Can you work these out from the model? Positions are in its coordinate system, mm. Face numbers are marked on the shaded views. A direction names the side the tool comes from. Coordinates: 2 decimals unless noted, no trailing zeros. Order: outer loops, then holes, each group sorted by start corner. A loop starts at its lowest first (then second) coordinate and runs counter-clockwise, first axis right, second up. Notation, with made-up numbers: (56, 0.25) - (64, 0.25) arc R21 cw to (64, 31.25) - close; hole circle Ø1 at (68, -7.5). An arc over 180 degrees is marked (long way). Return JSON: item names as keys, results as strings. Group by question number.
1) If I drill on line 1 along X through (y, z) = (0.85, 2.5); line 2 along Z through (x, y) = (12.75, 6.5); line 3 along Y through (x, z) = (11.5, 7.75), over which ranges is the centre line in solid material (lowest first)?
2) Imagine slicing it at D-D (y = 4.5). Write out the boundary of the cut face in (x, z), and give its area (3 significant figures).
3) If we mould it in two halves opening along X, with no side actions, what happens to the marked faces 3, 4 and 5? For each: pulls with the +X half, pulls with the -X half, needs draft (parallel to the pull), parting line crosses it, or undercut.
4) Imagine slicing it at C-C (x = 12.5). Write out the boundary of the cut face in (y, z).
5) Which directions (+Z, -Z, +X, -X, +Y, -Y) give clear straight access to the entire face, cutting with the end or side of a thin tool? Please do the marked faces 1 and 2.
6) Imagine slicing it at A-A (z = 2.5). Write out the boundary of the cut face in (x, y).
7) For pin 1 Ø6.5 at (x, z) = (10.5, 5.5) entering from -Y; pin 2 Ø7.5 at (x, y) = (8.5, 6) entering from -Z; pin 3 Ø0.5 at (y, z) = (-0.5, 11) entering from +X; pin 4 Ø2.5 at (x, z) = (15.5, 2.5) entering from -Y, each with a flat end and sliding along its axis, tell me the tip position at first contact or that it passes through.
8) Imagine slicing it at B-B (x = 15.5). Write out the boundary of the cut face in (y, z).
```python
from build123d import *

# Parameters (mm, degrees)
SKETCH_1_W      = 18
SKETCH_1_H      = 13
SKETCH_1_R      = 1.5
EXTRUDE_1_DEPTH = 1.6
SKETCH_2_W      = 15
SKETCH_2_H      = 1.5
EXTRUDE_2_DEPTH = 1
SKETCH_3_W      = 15.814161569
SKETCH_3_H      = 0.898910236
EXTRUDE_3_DEPTH = 15


with BuildPart() as part:
    # 草图1 → 凸台-拉伸1 (new body)
    with BuildSketch(Plane(origin=(0, 0, 0), x_dir=(1, 0, 0), z_dir=(0, 1, 0))):
        with Locations((9, -6.5)):
            Rectangle(SKETCH_1_W, SKETCH_1_H)
        with Locations(Location((2.5, -2.5, 0), (0, 0, 270))):
            Circle(SKETCH_1_R, mode=Mode.SUBTRACT)
        with Locations(Location((15.5, -2.5, 0), (0, 0, 270))):
            Circle(SKETCH_1_R, mode=Mode.SUBTRACT)
    extrude(amount=EXTRUDE_1_DEPTH)

    # 草图2 → 凸台-拉伸2 (add)
    with BuildSketch(Plane.XZ):
        with Locations((9, 11.25)):
            Rectangle(SKETCH_2_W, SKETCH_2_H)
    extrude(amount=EXTRUDE_2_DEPTH)

    # 草图3 → 凸台-拉伸3 (add)
    with BuildSketch(Plane(origin=(0, 1.6, 0), x_dir=(1, 0, 0), z_dir=(0, 1, 0))):
        with Locations((8.933414057, -11.968370606)):
            Rectangle(SKETCH_3_W, SKETCH_3_H)
    extrude(amount=EXTRUDE_3_DEPTH)


solid = part.part
```
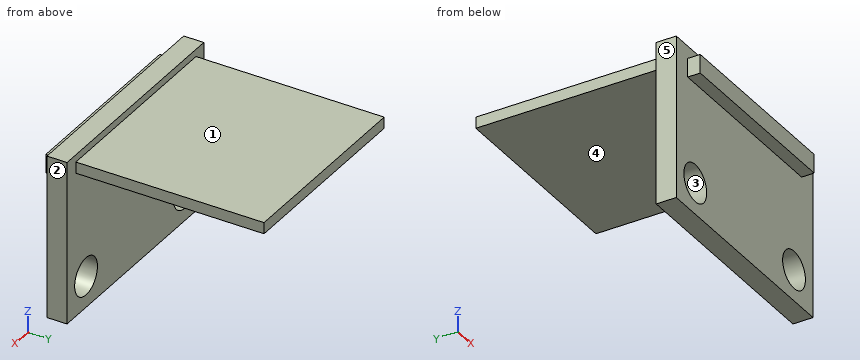
Calculated:
{
 "1": {"line 1": "0 to 1, 4 to 14, 17 to 18", "line 2": "11.52 to 12.42", "line 3": "0 to 1.6"},
 "2": {"outline": "(1.03, 11.52) - (16.84, 11.52) - (16.84, 12.42) - (1.03, 12.42) - close", "area": "14.2 mm2"},
 "3": {"face 3": "undercut", "face 4": "needs draft", "face 5": "pulls with the -X half"},
 "4": {"outline": "(-1, 10.5) - (0, 10.5) - (0, 0) - (1.6, 0) - (1.6, 11.52) - (16.6, 11.52) - (16.6, 12.42) - (1.6, 12.42) - (1.6, 13) - (0, 13) - (0, 12) - (-1, 12) - close"},
 "5": {"face 1": "+Z, +X, -X, +Y", "face 2": "+Z, -Z, +X, +Y, -Y"},
 "6": {"outline": "(0, 0) - (1, 0) - (1, 1.6) - (0, 1.6) - close; (4, 0) - (14, 0) - (14, 1.6) - (4, 1.6) - close; (17, 0) - (18, 0) - (18, 1.6) - (17, 1.6) - close"},
 "7": {"pin 1": "y = 0", "pin 2": "z = 11.52", "pin 3": "x = 16.5", "pin 4": "through"},
 "8": {"outline": "(-1, 10.5) - (0, 10.5) - (0, 4) - (1.6, 4) - (1.6, 11.52) - (16.6, 11.52) - (16.6, 12.42) - (1.6, 12.42) - (1.6, 13) - (0, 13) - (0, 12) - (-1, 12) - close; (0, 0) - (1.6, 0) - (1.6, 1) - (0, 1) - close"}
}
